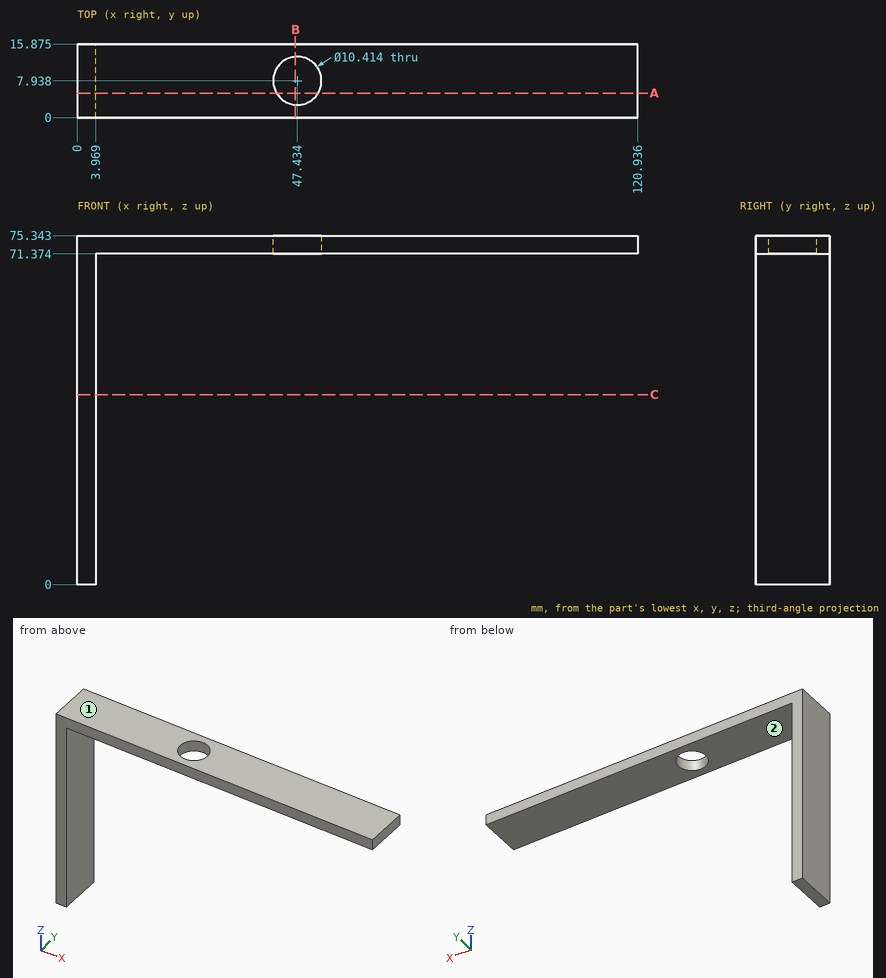
Geometry: see drawing. Coordinates: mm, zero at the bounding-box minimum. A direction names the side the tool comes from. Round coordinates to 2 decimals unless told otherwise and drop trailing zeros. Order: outer loops, then holes, each group sorted by start corner. A loop starts at its lowest first (then second) coordinate and runs counter-clockwise, first axis right, second up. Notation, with made-up numbers: (-37, -23) - (-16, -23) arc R22 cw to (-16, -9) - close; hole circle Ø2 at (54, 68). An arc over 180 degrees is marked (long way). Use a Markdown table: item, result. Add a question column.
1. Section query A-A (y = 5.25). Return the cut outline in (x, z) (1 decimal).
2. Set-up query: the marked faces 1 and 2. Return all of +Z, -Z, +X, -X, +Y, -Y with unobstructed straight access to the full face (end or side cutting, diameter ignored); none if empty.
3. First-contact query: pin 1 (4 mm diameter, centred on y = 10.5, z = 47, fed in from +X); pin 2 (5 mm diameter, centred on y = 8, z = 43, fed in from -X). Flat tips, straight axial feed; report the tip coordinate or a pass-through.
4. Section query B-B (x = 47). Return the cut outline in (y, z) (1 decimal).
5. Line query: probe 1 along X at (y, z) = (9.25, 26.5); probe 2 along Z at (x, y) = (115.5, 9.75) (1 decimal). Output: solid intervals per line, ascending.
6. Section query C-C (z = 41). Return the cut outline in (x, y) (1 decimal), then the cut area to 3 significant figures.
Derived:
| question | item | result |
|---|---|---|
| 1 | outline | (0, 0) - (4, 0) - (4, 71.4) - (43, 71.4) - (43, 75.3) - (0, 75.3) - close; (51.9, 71.4) - (120.9, 71.4) - (120.9, 75.3) - (51.9, 75.3) - close |
| 2 | face 1 | +Z, +X, -X, +Y, -Y |
| 2 | face 2 | -Z, +X, +Y, -Y |
| 3 | pin 1 | x = 3.97 |
| 3 | pin 2 | x = 0 |
| 4 | outline | (0, 71.4) - (2.7, 71.4) - (2.7, 75.3) - (0, 75.3) - close; (13.1, 71.4) - (15.9, 71.4) - (15.9, 75.3) - (13.1, 75.3) - close |
| 5 | probe 1 | 0 to 3.97 |
| 5 | probe 2 | 71.4 to 75.3 |
| 6 | outline | (0, 0) - (4, 0) - (4, 15.9) - (0, 15.9) - close |
| 6 | area | 63.0 mm2 |
